Read the model definition and answer for the solid it produces. Units are mm, in the model's axes. Coordinates: 2 decimals unless noted, no trailing zeros. Order: outer loops, then holes, each group sorted by start corner. A loop starts at its lowest first (then second) coordinate and runs counter-clockwise, first axis right, second up.
```python
from build123d import *

# Parameters (mm, degrees)
F1_DEPTH    = 25.4
F2_T1_DEPTH = 15.3225079539
F2_T3_DEPTH = 16.775320589
F2_T6_ANGLE = 87.0348581142
F2_T8_ANGLE = 103.9234369613
F3_R        = 1.2082658068
F4_DEPTH    = 25.4


# Not quite as in the source:
# - a fillet or chamfer that OpenCascade refuses, or shapes differently, is made with other operations: its cross-section is extruded or revolved along the edge and cut away or added


with BuildPart() as f1:
    # F0 (on Top) → F1 (new body)
    with BuildSketch(Plane.XY):
        with BuildLine():
            ThreePointArc((-7.752480221, -10.059276834), (-4.8810304794, -8.8387254095), (-2.3312001475, -7.0405778413))
            Line((-2.3312001475, -7.0405778413), (-4.1826744651, -3.1376440612))
            Line((-4.1826744651, -3.1376440612), (-12.0026959047, -4.1503362537))
            ThreePointArc((-12.0026959047, -4.1503362537), (-10.3099777223, -7.4158181858), (-7.752480221, -10.059276834))
        make_face()
        with BuildLine():
            ThreePointArc((-1.4857464298, -12.5192106342), (-1.6518399037, -10.7309962936), (-1.4257026774, -8.9493791841))
            Line((-1.4257026774, -8.9493791841), (-2.3312001475, -7.0405778413))
            ThreePointArc((-2.3312001475, -7.0405778413), (-4.8810304794, -8.8387254095), (-7.752480221, -10.059276834))
            ThreePointArc((-7.752480221, -10.059276834), (-4.8332265428, -11.7443569933), (-1.5735123086, -12.6021450164))
            Line((-1.5735123086, -12.6021450164), (-1.4857464298, -12.5192106342))
        make_face()
    extrude(amount=F1_DEPTH)

    # F2: fillet of radius 1.778 on 4 edges, made by hand

    # F2_s2 → F2_t1 (cut)
    with BuildSketch(Plane(origin=(5.1087634899, -10.7693449534, 0), x_dir=(0, 0, 1), z_dir=(-0.4285998257, 0.9034944324, 0))):
        with BuildLine():
            ThreePointArc((23.622, -5.1238167896), (24.8792358569, -5.6445809326), (25.4, -6.9018167896))
            Line((25.4, -6.9018167896), (25.4, -5.1238167896))
            Line((25.4, -5.1238167896), (23.622, -5.1238167896))
        make_face()
    extrude(amount=F2_T1_DEPTH, mode=Mode.SUBTRACT)

    # F2_s4 → F2_t3 (cut)
    with BuildSketch(Plane(origin=(-0.1051193903, -0.0136129532, 0), x_dir=(0, 0, 1), z_dir=(-0.9917188973, -0.1284275232, 0))):
        with BuildLine():
            ThreePointArc((23.622, -2.5744903868), (24.8792358569, -3.0952545299), (25.4, -4.3524903868))
            Line((25.4, -4.3524903868), (25.4, -2.5744903868))
            Line((25.4, -2.5744903868), (23.622, -2.5744903868))
        make_face()
    extrude(amount=F2_T3_DEPTH, mode=Mode.SUBTRACT)

    # F2_s5 → F2_t6 (revolve, cut)
    with BuildSketch(Plane(origin=(8.4191230763, -9.1705520677, 0), x_dir=(0, 0, 1), z_dir=(0.6762824344, -0.7366424295, 0))):
        with BuildLine():
            ThreePointArc((23.622, 10.7336378697), (24.8792358569, 11.2544020127), (25.4, 12.5116378697))
            Line((25.4, 12.5116378697), (25.4, 10.7336378697))
            Line((25.4, 10.7336378697), (23.622, 10.7336378697))
        make_face()
    revolve(axis=Axis((6.5687949782, -10.8692655012, 25.4), (0, 0, -1)), revolution_arc=F2_T6_ANGLE, mode=Mode.SUBTRACT)

    # F2_s7 → F2_t8 (revolve, cut)
    with BuildSketch(Plane(origin=(0, 0, 0), x_dir=(0, 0, 1), z_dir=(0.017156123, 0.9998528229, 0))):
        with BuildLine():
            ThreePointArc((23.622, -12.7), (24.8792358569, -12.1792358569), (25.4, -10.922))
            Line((25.4, -10.922), (25.4, -12.7))
            Line((25.4, -12.7), (23.622, -12.7))
        make_face()
    revolve(axis=Axis((0, 0, 25.4), (0, 0, 1)), revolution_arc=F2_T8_ANGLE, mode=Mode.SUBTRACT)

    # F3 (on face) → F4 (cut)
    with BuildSketch(Plane(origin=(-4.6293399422, -2.1960669829, 0), x_dir=(-0.4285998257, 0.9034944324, 0), z_dir=(0.9034944324, 0.4285998257, 0))):
        with Locations((-4.8675471917, 19.804911688)):
            Circle(F3_R)
    extrude(amount=-F4_DEPTH, mode=Mode.SUBTRACT)


solid = f1.part
```
1) A cutting plane is placed at A-A, the plane z = 21.5. Determine the outline of the cut face in (x, y).
A:
outline: (-12, -4.15) arc R12.7 ccw to (-1.57, -12.6) - (-1.49, -12.52) arc R8.22 cw to (-1.43, -8.95) - (-4.18, -3.14) - close
2) Straight lines are drawn through the part: line 1 (Z direction, x = -4, y = -7.75); line 2 (Z direction, x = -3.5, y = -6); line 3 (Y direction, x = -4.5, z = 2.5). For each, find the intervals that lie inside material, in ascending order.
A:
line 1: z = 0 to 18.67, 20.94 to 25.4
line 2: z = 0 to 19.05, 20.56 to 24.96
line 3: y = -11.88 to -3.18
3) Determine the mould class of faces 1 (the cylindrical face through (-7.973, -4.14, 24.865)), 2 (the flat face through (-6, -7, 25.4)), 3 (the cylindrical face through (-1.652, -10.756, 11.646)) for opening direction Y: pulls with the +Y half, pulls with the -Y half, needs draft (parallel to the pull), parting line crosses it, or undercut.
A:
face 1: pulls with the +Y half
face 2: needs draft
face 3: undercut
4) Flat-ended cylindrical pins translate along their axes: pin 1 Ø5 at (y, z) = (-9, 6.5) entering from +X; pin 2 Ø1 at (x, z) = (-3, 11.5) entering from -Y; pin 3 Ø2 at (x, z) = (-10.5, 19.5) entering from +Y; pin 4 Ø5 at (x, z) = (-7, 15) entering from -Y. Find the tip coordinate at first contact, or state that the pin passes through.
A:
pin 1: stops at x = -1.43
pin 2: stops at y = -12.45
pin 3: stops at y = -3.83
pin 4: stops at y = -11.88
